```python
from build123d import *

# Parameters (mm, degrees)
CROQUIS1_W              = 25
CROQUIS1_H              = 3
SALIENTE_EXTRUIR1_DEPTH = 195
CROQUIS2_R              = 4.25
CORTAR_EXTRUIR1_DEPTH   = 195
CROQUIS3_W              = 4
CROQUIS3_H              = 25
SALIENTE_EXTRUIR2_DEPTH = 195
SALIENTE_EXTRUIR3_START = 1
CROQUIS4_W              = 29
CROQUIS4_H              = 195
CROQUIS4_R              = 4.25
SALIENTE_EXTRUIR3_DEPTH = 1
CROQUIS5_W              = 80.668780501
CROQUIS5_H              = 25.5
CORTAR_EXTRUIR2_DEPTH   = 30
CROQUIS6_R              = 4.25
CORTAR_EXTRUIR3_DEPTH   = 30
CROQUIS7_R              = 4.25
SALIENTE_EXTRUIR4_DEPTH = 4


with BuildPart() as part:
    # Croquis1 → Saliente-Extruir1 (new body)
    with BuildSketch(Plane(origin=(0, 0, 0), x_dir=(1, 0, 0), z_dir=(0, 1, 0))):
        with Locations((12.5, -1.5)):
            Rectangle(CROQUIS1_W, CROQUIS1_H)
    extrude(amount=SALIENTE_EXTRUIR1_DEPTH)

    # Croquis2 → Cortar-Extruir1 (cut)
    with BuildSketch(Plane.XY.offset(3)):
        with Locations((18.25, 180)):
            Circle(CROQUIS2_R)
        with Locations((18.25, 97.5)):
            Circle(CROQUIS2_R)
        with Locations((18.25, 15)):
            Circle(CROQUIS2_R)
    extrude(amount=-CORTAR_EXTRUIR1_DEPTH, mode=Mode.SUBTRACT)

    # Croquis3 → Saliente-Extruir2 (add)
    with BuildSketch(Plane(origin=(0, 195, 0), x_dir=(1, 0, 0), z_dir=(0, 1, 0))):
        with Locations((-2, 9.5)):
            Rectangle(CROQUIS3_W, CROQUIS3_H)
    extrude(amount=-SALIENTE_EXTRUIR2_DEPTH)

    # Croquis4 → Saliente-Extruir3 (add)
    with BuildSketch(Plane.XY.offset(3).offset(SALIENTE_EXTRUIR3_START)):
        with Locations((10.5, 97.5)):
            Rectangle(CROQUIS4_W, CROQUIS4_H)
        with Locations((18.25, 15)):
            Circle(CROQUIS4_R, mode=Mode.SUBTRACT)
        with Locations((18.25, 97.5)):
            Circle(CROQUIS4_R, mode=Mode.SUBTRACT)
        with Locations((18.25, 180)):
            Circle(CROQUIS4_R, mode=Mode.SUBTRACT)
    extrude(amount=-SALIENTE_EXTRUIR3_DEPTH)

    # Croquis5 → Cortar-Extruir2 (cut)
    with BuildSketch(Plane.XY.offset(4)):
        with Locations((-15.334390251, 182.25)):
            Rectangle(CROQUIS5_W, CROQUIS5_H)
    extrude(amount=-CORTAR_EXTRUIR2_DEPTH, mode=Mode.SUBTRACT)

    # Croquis6 → Cortar-Extruir3 (cut)
    with BuildSketch(Plane.XY.offset(4)):
        with Locations((18.25, 154.5)):
            Circle(CROQUIS6_R)
    extrude(amount=-CORTAR_EXTRUIR3_DEPTH, mode=Mode.SUBTRACT)

    # Croquis7 → Saliente-Extruir4 (add)
    with BuildSketch(Plane.XY.offset(4)):
        with Locations((18.25, 97.5)):
            Circle(CROQUIS7_R)
    extrude(amount=-SALIENTE_EXTRUIR4_DEPTH)


solid = part.part
```
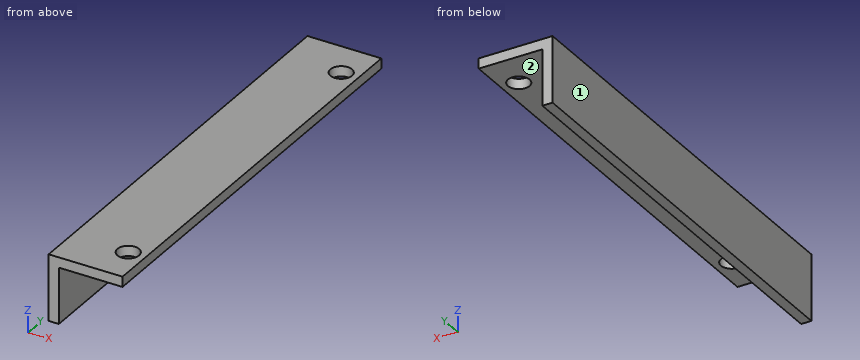
Can you work these out from the model? Positions are in its coordinate system, mm. Face numbers are marked on the shaded views. A direction names the side the tool comes from. Give positions to 0.01 mm unless a question says otherwise; leave off trailing zeros. Write each loop counter-clockwise with the first axis right and the second up, starting at its lowest first coordinate (ties: lowest second). Pieces come first, ordered by that corner, then holes. Notation, with made-up numbers: (22, 21) -> (40, 21) arc R36 cw to (40, 58) -> close; hole circle Ø9 at (60.25, 39). An arc over 180 degrees is marked (long way). Write item = value, one per line.
(1) Suppose I cut it at B-B on y = 154.5. Write out the boundary of the cut face in (x, z), then the cut area to 3 significant figures.
Worked out:
outline = (-4, -22) -> (0, -22) -> (0, 0) -> (14, 0) -> (14, 4) -> (-4, 4) -> close; (22.5, 0) -> (25, 0) -> (25, 4) -> (22.5, 4) -> close
area = 170 mm^2
(2) I need wall thicknesses on probe 1 along Y at (x, z) = (18.25, 1.9); probe 2 along Z at (x, y) = (19.5, 35.5); probe 3 along X at (y, z) = (132.5, -11). Which ranges of each line are inside material? Lowest first, please. Write a range as from..to.
Worked out:
probe_1 = 0..10.75, 19.25..150.25, 158.75..169.5
probe_2 = 0..4
probe_3 = -4..0
(3) I'm going to push flat-ended pins straight in: P1, Ø10, axis at y = 100.5, z = -8, coming from the +X side; P2, Ø11, axis at x = 18.25, y = 15, coming from the +Z side; P3, Ø10, axis at x = 13.5, z = -8.5, coming from the -Y side; P4, Ø7.5, axis at x = 17.5, y = 68, coming from the -Z side. Where does each tip first touch, or does it pass through?
Worked out:
P1 = 0
P2 = 4
P3 = through
P4 = 0
(4) Suppose I cut it at D-D on x = 11.25. Write out the boundary of the cut face in (y, z), then the cut area to 3 significant figures.
Worked out:
outline = (0, 0) -> (169.5, 0) -> (169.5, 4) -> (0, 4) -> close
area = 678 mm^2
(5) For the marked faces 1 and 2, which set-ups out of +Z, -Z, +X, -X, +Y, -Y let a thin tool reach every point of the face, with its end or its side?
Worked out:
face_1 = +Z, -Z, -X, +Y, -Y
face_2 = -Z, +X, +Y, -Y
(6) Suppose I cut it at C-C on y = 91.5. Write out the boundary of the cut face in (x, z).
Worked out:
outline = (-4, -22) -> (0, -22) -> (0, 0) -> (25, 0) -> (25, 4) -> (-4, 4) -> close
(7) Suppose I cut it at A-A on x = 18.25. Write out the boundary of the cut face in (y, z), then the cut area to 3 significant figures.
Worked out:
outline = (0, 0) -> (10.75, 0) -> (10.75, 4) -> (0, 4) -> close; (19.25, 0) -> (150.25, 0) -> (150.25, 4) -> (19.25, 4) -> close; (158.75, 0) -> (169.5, 0) -> (169.5, 4) -> (158.75, 4) -> close
area = 610 mm^2
